Could you check a few things on this drawing? It's one solid part, dimensions in mm from its lowest x, y, z. Coordinates: 2 decimals unless noted, no trailing zeros. Order: outer loops, then holes, each group sorted by start corner. A loop starts at its lowest first (then second) coordinate and runs counter-clockwise, first axis right, second up. Notation, with made-up numbers: M 52.5,-25.5 L 76.5,-25.5 A3 ccw 76.5,-20.5 Z; hole C -26.5,68.5 d3. An arc over 180 degrees is marked long. Write item = value, one per line. Start each with the question number.
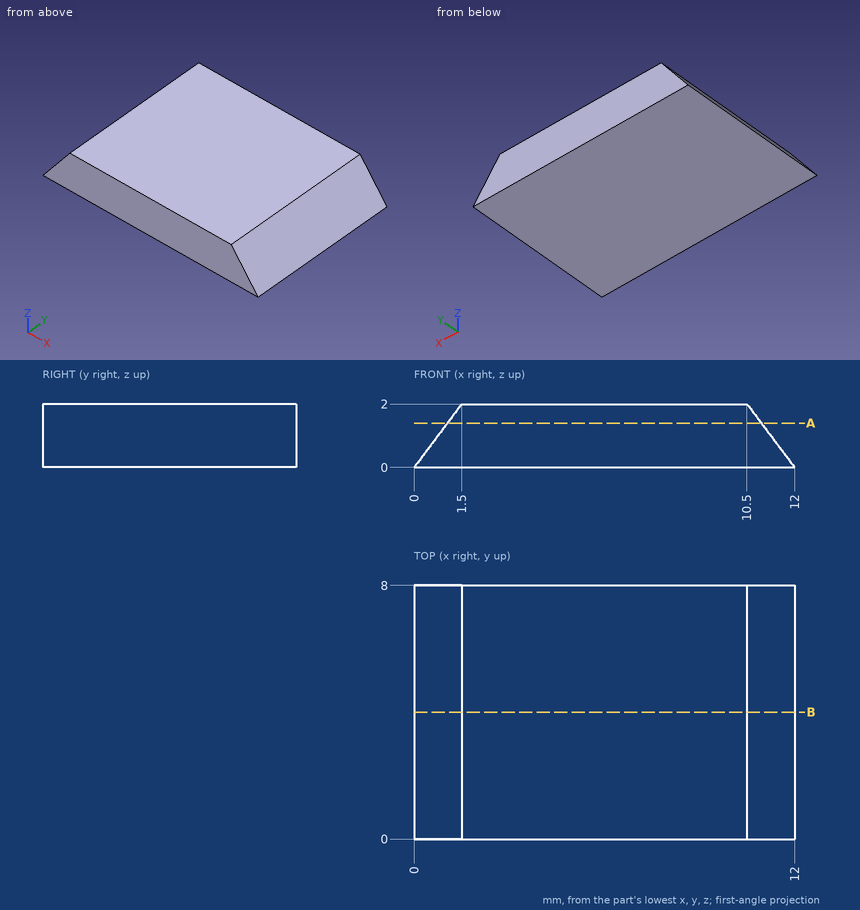
(1) Imagine slicing it at A-A on z = 1.4. List the corners of the cut face in (x, y) for me.
(2) Please list where these lines run through material, in increasing order: probe 1 along X at (y, z) = (5, 0.1) (3 decimals); probe 2 along X at (y, z) = (1.25, 0.5) (3 decimals); probe 3 along Z at (x, y) = (11, 0.5). Write a range as from..to.
(3) Will this pin go through, and if not, where does the flat tip stop? P1, Ø1, axis at y = 3.5, z = 1.5, coming from the -X side.
(4) Imagine slicing it at B-B on y = 4. List the corners of the cut face in (x, z) for me.
Response:
q1.outline = M 1.05,0 L 10.95,0 L 10.95,8 L 1.05,8 Z
q2.probe_1 = 0.075..11.925
q2.probe_2 = 0.375..11.625
q2.probe_3 = 0..1.33
q3.P1 = 0.75
q4.outline = M 0,0 L 12,0 L 10.5,2 L 1.5,2 Z
